Autodesk Inventor part; units mm, degrees
ref_plane "YZ Plane" through (0, 0, 0) normal (1, 0, 0) x (0, 1, 0)
ref_plane "XZ Plane" through (0, 0, 0) normal (0, 1, 0) x (-1, 0, 0)
ref_plane "XY Plane" through (0, 0, 0) normal (0, 0, 1) x (1, 0, 0)
sketch "Sketch1" plane through (0, 0, 0) normal (0, 0, 1) x (1, 0, 0)
  line L0 (0, 0) -> (15.5, 0)
  line L1 (15.5, 0) -> (15.5, 3)
  line L2 (15.5, 3) -> (0, 3)
  line L3 (0, 3) -> (0, 0)
  line L4 (15.5, 0) -> (18.5, 0)
  line L5 (18.5, 0) -> (18.5, 5)
  line L6 (18.5, 5) -> (15.5, 5)
  line L7 (15.5, 5) -> (15.5, 0)
  line L8 (0, 0) -> (18.5, 0)
  dimension "d0" = 5
  dimension "d1" = 3
  dimension "d2" = 15.5
  dimension "d3" = 3
revolve "Revolution1" add sketch "Sketch1" angle 360 about axis through (15.5, 0, 0) along (1, 0, 0)
fillet "Fillet1" radius 0.5 1 edges at (15.5, -3, 0)
chamfer "Chamfer1" distance 0.5 angle 45 2 edges at (0, -3, 0) (15.5, -5, 0)
sketch "Sketch2" plane through (18.5, 0, 0) normal (-1, 0, 0) x (0, 0, 1)
  circle A0 centre (0, 0) radius 3
  point P0 (0, 0)
hole "Hole1" at (18.5, 0, 0) direction (-1, 0, 0) diameter 2.459 end through all
properties part number "Pancake_Lever Mount Piece" material "Aluminum 6061"
Input: part model. Units: mm. Frame: model coordinates. A direction names the side the tool comes from. Coordinates: 2 decimals unless noted, no trailing zeros. Write each loop counter-clockwise with the first axis right and the second up, starting at its lowest first coordinate (ties: lowest second). Pieces come first, ordered by that corner, then holes. Notation, with made-up numbers: M 71,-36 L 124,-36 A8 ccw 124,-24 Z; hole C 13,-27 d8. An arc over 180 degrees is marked long. Answer as a JSON object with one key per item and string values. Group by question number.
(1) Set-up query: faces 4 (the face through (0, 1, 1)), 5 (the face through (8, -3, 0)). Return all of +Z, -Z, +X, -X, +Y, -Y with unobstructed straight access to the full face (end or side cutting, diameter ignored); none if empty.
(2) Section A-A on z = 0. Output: boundary loops of the cut face in (x, y), plus the area to 3 significant figures.
(3) Section C-C on x = 12. Output: boundary loops of the cut face in (y, z).
(4) Mould query, pull axis Z, two halves, no side actions, for faces 1 (the face through (17.23, -1.08, 4.88)), 2 (the face through (18.5, 1, -1)), 3 (the face through (9.12, 0.748, 0.976)). Classes: pulls with the +Z half, pulls with the -Z half, needs draft (parallel to the pull), parting line crosses it, or undercut.
(5) Contact query for flat-ended pins moving along their axis: P1, Ø1.5, axis at x = 4.5, z = 1, coming from the -Y side; P2, Ø1.5, axis at x = 15.5, z = 3, coming from the -Y side; P3, Ø3, axis at x = 13, y = 1, coming from the +Z side. Output: stop coordinate, or through.
(6) Ray query, line 1 along Z through (x, y) = (13.75, 0); line 2 along Z through (x, y) = (11.25, -1); line 3 along X through (y, z) = (0.25, 4.25). Return the intervals inside material, ascending. Write a range as [from, to].
Result set:
{
 "1": {"face 4": "+Z, -Z, -X, +Y, -Y", "face 5": "-X"},
 "2": {"outline": "M 0,-2.5 L 0.5,-3 L 15,-3 A0.5 cw 15.5,-3.5 L 15.5,-4.5 L 16,-5 L 18.5,-5 L 18.5,-1.23 L 0,-1.23 Z; M 0,1.23 L 18.5,1.23 L 18.5,5 L 16,5 L 15.5,4.5 L 15.5,3.5 A0.5 cw 15,3 L 0.5,3 L 0,2.5 Z", "area": "77.1 mm2"},
 "3": {"outline": "C 0,0 d6; hole C 0,0 d2.46"},
 "4": {"face 1": "parting line crosses it", "face 2": "needs draft", "face 3": "undercut"},
 "5": {"P1": "stops at y = -2.99", "P2": "stops at y = -4.36", "P3": "stops at z = 3"},
 "6": {"line 1": "z = [-3, -1.23], [1.23, 3]", "line 2": "z = [-2.83, -0.72], [0.72, 2.83]", "line 3": "x = [15.5, 18.5]"}
}
